from build123d import *

# Parameters (mm, degrees)
SALIENTE_EXTRUIR1_DEPTH = 4


with BuildPart() as part:
    # Croquis1 → Saliente-Extruir1 (new body)
    with BuildSketch(Plane.XY):
        with BuildLine():
            Line((-48.365211809, -20.854133368), (-51.695211809, -20.854133368))
            ThreePointArc((-51.695211809, -20.854133368), (-55.937852496, -19.096774055), (-57.695211809, -14.854133368))
            Line((-57.695211809, -14.854133368), (-57.695211809, 43.145866632))
            ThreePointArc((-57.695211809, 43.145866632), (-55.937852496, 47.388507319), (-51.695211809, 49.145866632))
            Line((-51.695211809, 49.145866632), (-48.365211809, 49.145866632))
            Line((-48.365211809, 49.145866632), (-48.365211809, 53.145866632))
            Line((-48.365211809, 53.145866632), (-43.365211809, 53.145866632))
            Line((-43.365211809, 53.145866632), (-43.365211809, 49.145866632))
            Line((-43.365211809, 49.145866632), (-27.235211809, 49.145866632))
            Line((-27.235211809, 49.145866632), (-27.235211809, 47.645866632))
            Line((-27.235211809, 47.645866632), (-29.735211809, 47.645866632))
            Line((-29.735211809, 47.645866632), (-29.735211809, 44.645866632))
            Line((-29.735211809, 44.645866632), (-20.735211809, 44.645866632))
            Line((-20.735211809, 44.645866632), (-20.735211809, 47.645866632))
            Line((-20.735211809, 47.645866632), (-23.235211809, 47.645866632))
            Line((-23.235211809, 47.645866632), (-23.235211809, 49.145866632))
            Line((-23.235211809, 49.145866632), (-19.225211809, 49.145866632))
            ThreePointArc((-19.225211809, 49.145866632), (-14.982571122, 47.388507319), (-13.225211809, 43.145866632))
            Line((-13.225211809, 43.145866632), (-13.225211809, -14.854133368))
            ThreePointArc((-13.225211809, -14.854133368), (-14.982571122, -19.096774055), (-19.225211809, -20.854133368))
            Line((-19.225211809, -20.854133368), (-30.315211809, -20.854133368))
            Line((-30.315211809, -20.854133368), (-30.315211809, -19.354133368))
            Line((-30.315211809, -19.354133368), (-27.815211809, -19.354133368))
            Line((-27.815211809, -19.354133368), (-27.815211809, -16.354133368))
            Line((-27.815211809, -16.354133368), (-36.815211809, -16.354133368))
            Line((-36.815211809, -16.354133368), (-36.815211809, -19.354133368))
            Line((-36.815211809, -19.354133368), (-34.315211809, -19.354133368))
            Line((-34.315211809, -19.354133368), (-34.315211809, -20.854133368))
            Line((-34.315211809, -20.854133368), (-43.365211809, -20.854133368))
            Line((-43.365211809, -20.854133368), (-43.365211809, -24.854133368))
            Line((-43.365211809, -24.854133368), (-48.365211809, -24.854133368))
            Line((-48.365211809, -24.854133368), (-48.365211809, -20.854133368))
        make_face()
        with BuildLine():
            Line((-47.695211809, 14.145866632), (-47.695211809, -8.854133368))
            ThreePointArc((-47.695211809, -8.854133368), (-47.109425371, -10.26834693), (-45.695211809, -10.854133368))
            Line((-45.695211809, -10.854133368), (-25.225211809, -10.854133368))
            ThreePointArc((-25.225211809, -10.854133368), (-23.810998246, -10.26834693), (-23.225211809, -8.854133368))
            Line((-23.225211809, -8.854133368), (-23.225211809, 37.145866632))
            ThreePointArc((-23.225211809, 37.145866632), (-23.810998246, 38.560080194), (-25.225211809, 39.145866632))
            Line((-25.225211809, 39.145866632), (-45.695211809, 39.145866632))
            ThreePointArc((-45.695211809, 39.145866632), (-47.109425371, 38.560080194), (-47.695211809, 37.145866632))
            Line((-47.695211809, 37.145866632), (-47.695211809, 14.145866632))
        make_face(mode=Mode.SUBTRACT)
    extrude(amount=SALIENTE_EXTRUIR1_DEPTH)


solid = part.part
Can you work these out from the model? Positions are in its coordinate system, mm. A direction names the side the tool comes from. Round coordinates to 2 decimals unless told otherwise and drop trailing zeros. Write each loop counter-clockwise with the first axis right and the second up, starting at its lowest first coordinate (ties: lowest second). Pieces come first, ordered by that corner, then holes. Notation, with made-up numbers: (73.25, 27.5) -> (106.25, 27.5) arc R12 ccw to (106.25, 50.5) -> close; hole circle Ø3 at (5, 20.25). An arc over 180 degrees is marked (long way). Use one line per item in the form item = value. Start each with the question number.
Q1. Imagine slicing it at B-B (x = -29). Please give me the cut outline in (y, z), then the cut area to 3 significant figures.
Q2. Imagine slicing it at D-D (x = -16.5). Please give me the cut outline in (y, z), then the cut area to 3 significant figures.
Q3. We'd pull the mould along Y, two halves only. Please class faces 1 (the face through (-48.365, -23, 2)), 2 (the face through (-23.796, 38.544, 1.972)), 3 (the face through (-55.984, 47.342, 1.972)): +Y half, -Y half, draft (parallel to the pull), parting line (faces both ways), or undercut.
Q4. Imagine slicing it at A-A (x = -22). Please give me the cut outline in (y, z), then the cut area to 3 significant figures.
Q5. Imagine slicing it at C-C (y = 33). Please give me the cut outline in (x, z).
Q6. I'm going to push flat-ended pins straight in: P1, Ø2, axis at x = -34.5, z = 1, coming from the -Y side; P2, Ø1.6, axis at y = 48, z = 2, coming from the -X side; P3, Ø1, axis at x = -32, z = 2.5, coming from the -Y side. Where does each tip first touch, or does it pass through?
Q7. If I drill on probe 1 along Y at (x, z) = (-30, 1.8); probe 2 along X at (y, z) = (9, 3.1); probe 3 along Y at (x, z) = (-44, 1.45), over which ranges is the centre line in solid material (lowest first)? Write a range as [from, to].
Q8. Which directions (+Z, -Z, +X, -X, +Y, -Y) give clear straight access to the entire face, cutting with the end or side of a thin tool? Please do faces 4 (the face through (-35, 39.146, 2)), 5 (the face through (-21, 49.146, 2)), 6 (the face through (-23.235, 48, 2)).
Worked out:
q1.outline = (-20.85, 0) -> (-19.35, 0) -> (-19.35, 4) -> (-20.85, 4) -> close; (-16.35, 0) -> (-10.85, 0) -> (-10.85, 4) -> (-16.35, 4) -> close; (39.15, 0) -> (44.65, 0) -> (44.65, 4) -> (39.15, 4) -> close; (47.65, 0) -> (49.15, 0) -> (49.15, 4) -> (47.65, 4) -> close
q1.area = 56.0 mm^2
q2.outline = (-20.2, 0) -> (48.49, 0) -> (48.49, 4) -> (-20.2, 4) -> close
q2.area = 275 mm^2
q3.face_1 = draft
q3.face_2 = undercut
q3.face_3 = +Y half
q4.outline = (-20.85, 0) -> (44.65, 0) -> (44.65, 4) -> (-20.85, 4) -> close; (47.65, 0) -> (49.15, 0) -> (49.15, 4) -> (47.65, 4) -> close
q4.area = 268 mm^2
q5.outline = (-57.7, 0) -> (-47.7, 0) -> (-47.7, 4) -> (-57.7, 4) -> close; (-23.23, 0) -> (-13.23, 0) -> (-13.23, 4) -> (-23.23, 4) -> close
q6.P1 = -20.85
q6.P2 = -56.12
q6.P3 = -16.35
q7.probe_1 = [-20.85, -19.35], [-16.35, -10.85], [39.15, 49.15]
q7.probe_2 = [-57.7, -47.7], [-23.23, -13.23]
q7.probe_3 = [-24.85, -10.85], [39.15, 53.15]
q8.face_4 = +Z, -Z
q8.face_5 = +Z, -Z, +X, +Y
q8.face_6 = +Z, -Z, +Y
